CAD build for the part. Positions are in the model's coordinates, mm. Coordinates: 2 decimals unless noted, no trailing zeros. Loops run counter-clockwise (first coordinate to the right, second up) from the corner with the lowest first, then second, coordinate; pieces in that order, holes last. Notation, with made-up numbers: (-32, 65.5) - (23, 65.5) arc R17 ccw to (23, 93.5) - close; hole circle Ø7 at (72, -29.5). An arc over 180 degrees is marked (long way). Put each result on its own line as item: value.
```python
from build123d import *

# Parameters (mm, degrees)
CROQUIS1_R              = 6.9
SALIENTE_EXTRUIR3_DEPTH = 5.38
CROQUIS4_OUTSIDE_W      = 19.848
CROQUIS4_OUTSIDE_H      = 19.848
CROQUIS4_OUTSIDE_R      = 6.5
CORTAR_EXTRUIR2_DEPTH   = 4
CORTAR_EXTRUIR3_REACH   = 13.143
CROQUIS5_R              = 4.8


with BuildPart() as part:
    # Croquis1 → Saliente-Extruir3 (new body)
    with BuildSketch(Plane.XY):
        Circle(CROQUIS1_R)
    extrude(amount=SALIENTE_EXTRUIR3_DEPTH)

    # Croquis4 outside → Cortar-Extruir2 (cut)
    with BuildSketch(Plane.XY.offset(5.38)):
        Rectangle(CROQUIS4_OUTSIDE_W, CROQUIS4_OUTSIDE_H)
        Circle(CROQUIS4_OUTSIDE_R, mode=Mode.SUBTRACT)
    extrude(amount=-CORTAR_EXTRUIR2_DEPTH, mode=Mode.SUBTRACT)

    # Croquis5 → Cortar-Extruir3 (cut, up to next)
    with BuildSketch(Plane.XY.offset(5.38), mode=Mode.PRIVATE) as cortar_extruir3_sk1:
        Circle(CROQUIS5_R)
    cortar_extruir3_tool1 = extrude(cortar_extruir3_sk1.sketch, amount=-CORTAR_EXTRUIR3_REACH, mode=Mode.PRIVATE) & part.part
    add(cortar_extruir3_tool1.solids().sort_by_distance((0, 0, 5.38))[0], mode=Mode.SUBTRACT)


solid = part.part
```
Q1. Slice it at A-A, the plane x = 0. Give the cut face in (y, z), then the cut area to 3 significant figures.
Determined:
outline: (-6.9, 0) - (-4.8, 0) - (-4.8, 5.38) - (-6.5, 5.38) - (-6.5, 1.38) - (-6.9, 1.38) - close; (4.8, 0) - (6.9, 0) - (6.9, 1.38) - (6.5, 1.38) - (6.5, 5.38) - (4.8, 5.38) - close
area: 19.4 mm2
Q2. Slice it at B-B, the plane y = -1.25. Give the cut face in (x, z).
Determined:
outline: (-6.79, 0) - (-4.63, 0) - (-4.63, 5.38) - (-6.38, 5.38) - (-6.38, 1.38) - (-6.79, 1.38) - close; (4.63, 0) - (6.79, 0) - (6.79, 1.38) - (6.38, 1.38) - (6.38, 5.38) - (4.63, 5.38) - close
Q3. Slice it at C-C, the plane z = 4.3. Give the cut face in (x, y), then the cut area to 4 significant figures.
Determined:
outline: circle Ø13 at (0, 0); hole circle Ø9.6 at (0, 0)
area: 60.35 mm2
Q4. Pin check, flat tip, straight feed: pin 1 Ø1 at (x, z) = (2.5, 3.5) entering from +Y. Stop position of the tip, or through.
Determined:
pin 1: y = 6.18
Q5. Slice it at D-D, the plane y = 6. Give the cut face in (x, z).
Determined:
outline: (-3.41, 0) - (3.41, 0) - (3.41, 1.38) - (2.5, 1.38) - (2.5, 5.38) - (-2.5, 5.38) - (-2.5, 1.38) - (-3.41, 1.38) - close
Q6. Wall check: L1, parallel to Y at x = 0, z = 2.55; L2, parallel to X at y = 3.75, z = 2.55; L3, parallel to Y at x = -1, z = 1.2. Give the ranges that are in metal, low to high. Write a range as from..to.
Determined:
L1: -6.5..-4.8, 4.8..6.5
L2: -5.31..-3, 3..5.31
L3: -6.83..-4.69, 4.69..6.83
Q7. Mould opens along X. For faces 1 (the cylindrical face through (2.58, 4.05, 2.73)), 2 (the cylindrical face through (-5.158, -3.955, 3.408)), 3 (the flat face through (6, -3, 1.38)) say: +X half, -X half, draft (parallel to the pull), parting line (faces both ways), or undercut.
Determined:
face 1: undercut
face 2: parting line
face 3: draft
